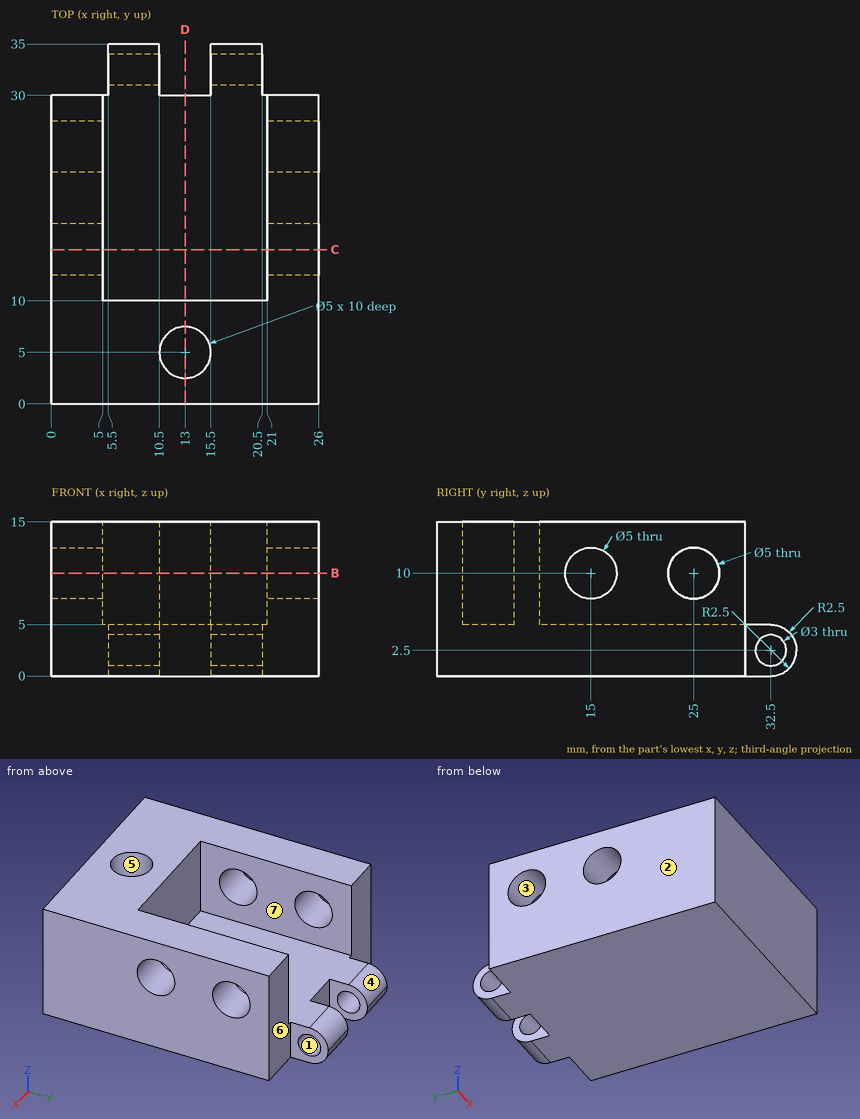
Could you check a few things on this drawing? It's one solid part, dimensions in mm from its lowest x, y, z. A direction names the side the tool comes from. Coordinates: 2 decimals unless noted, no trailing zeros. Write each loop counter-clockwise with the first axis right and the second up, starting at its lowest first coordinate (ties: lowest second). Pieces come first, ordered by that corner, then holes. Notation, with made-up numbers: (0, 2.25) - (9, 2.25) arc R11 cw to (9, 6.25) - close; hole circle Ø11 at (70, -21.5). An arc over 180 degrees is marked (long way). Write item = value, one per line.
1) Suppose I cut it at C-C on y = 15. Please give me the cut outline in (x, z), plus the area to 3 significant figures.
Result set:
outline = (0, 0) - (26, 0) - (26, 7.5) - (21, 7.5) - (21, 5) - (5, 5) - (5, 7.5) - (0, 7.5) - close; (0, 12.5) - (5, 12.5) - (5, 15) - (0, 15) - close; (21, 12.5) - (26, 12.5) - (26, 15) - (21, 15) - close
area = 180 mm2
2) Will these pins go through, and if not, where does the flat tip stop? pin 1 Ø3 at (x, z) = (7.5, 5) entering from -Y; pin 2 Ø8 at (x, y) = (13, 19.5) entering from +Z; pin 3 Ø1.5 at (y, z) = (33.5, 3.5) entering from -X; pin 4 Ø2.5 at (y, z) = (32.5, 2.5) entering from -X.
Result set:
pin_1 = 0
pin_2 = 5
pin_3 = 5.5
pin_4 = through
3) Please list where these lines run through material, in increasing order: line 1 (Y direction, x = 3.25, z = 10); line 2 (Y direction, x = 8, z = 2.5); line 3 (X direction, y = 24.5, z = 5.75). Write a range as [from, to].
Result set:
line_1 = [0, 12.5], [17.5, 22.5], [27.5, 30]
line_2 = [0, 31], [34, 35]
line_3 = [0, 5], [21, 26]
4) Suppose I cut it at D-D on x = 13. Please give me the cut outline in (y, z), plus the area to 3 significant figures.
Result set:
outline = (0, 0) - (30, 0) - (30, 5) - (10, 5) - (10, 15) - (7.5, 15) - (7.5, 5) - (2.5, 5) - (2.5, 15) - (0, 15) - close
area = 200 mm2
5) Suppose I cut it at B-B on z = 10. Please give me the cut outline in (x, y).
Result set:
outline = (0, 0) - (26, 0) - (26, 12.5) - (21, 12.5) - (21, 10) - (5, 10) - (5, 12.5) - (0, 12.5) - close; (0, 17.5) - (5, 17.5) - (5, 22.5) - (0, 22.5) - close; (0, 27.5) - (5, 27.5) - (5, 30) - (0, 30) - close; (21, 17.5) - (26, 17.5) - (26, 22.5) - (21, 22.5) - close; (21, 27.5) - (26, 27.5) - (26, 30) - (21, 30) - close; hole circle Ø5 at (13, 5)
6) For the marked faces 5, 6 and 7, which set-ups out of +Z, -Z, +X, -X, +Y, -Y let a thin tool reach every point of the face, with its end or its side?
Result set:
face_5 = +Z
face_6 = +Z, -Z, +X, +Y
face_7 = +Z, +Y
7) We'd pull the mould along Z, two halves only. Please class the marked faces 1, 2, 3 and 4: +Z half, -Z half, draft (parallel to the pull), parting line (faces both ways), or undercut.
Result set:
face_1 = undercut
face_2 = draft
face_3 = undercut
face_4 = +Z half
